Job drawing, mm, ordinate dimensions from the low corner. One solid piece. Give positions to 0.01 mm unless a question says otherwise; leave off trailing zeros. Write each loop counter-clockwise with the first axis right and the second up, starting at its lowest first coordinate (ties: lowest second). Pieces come first, ordered by that corner, then holes. Notation, with made-up numbers: (-18.75, 16) -> (1.25, 16) arc R22 cw to (1.25, 35) -> close; hole circle Ø2 at (-27.5, 83.25). An arc over 180 degrees is marked (long way). One line per question, with ' | ' between items. Start each with the question number.
(1) Band-saw the part on A-A, the plane z = 8. Give the cut face in (x, y).
(2) Band-saw the part on D-D, the plane x = 7. Give the cut face in (y, z), and give its area (3 significant figures).
(3) Pin check, flat tips, straight feed: P1, Ø2, axis at x = 4.5, y = 3.5, coming from the -Z side; P2, Ø2, axis at x = 32, y = 3.5, coming from the +Z side; P3, Ø4, axis at x = 11, z = 48, coming from the +Y side. Stop position of each tip, or through.
(4) Band-saw the part on C-C, the plane x = 11. Give the cut face in (y, z).
(5) Band-saw the part on B-B, the plane y = 1. Give the cut face in (x, z), and give its area (3 significant figures).
(6) Drill centre lines: probe 1 along Z at (x, y) = (27, 1.4); probe 2 along X at (y, z) = (0.45, 8); probe 3 along X at (y, z) = (3.75, 32). Where is each one in solid material? Low to high. Write a range as from..to.
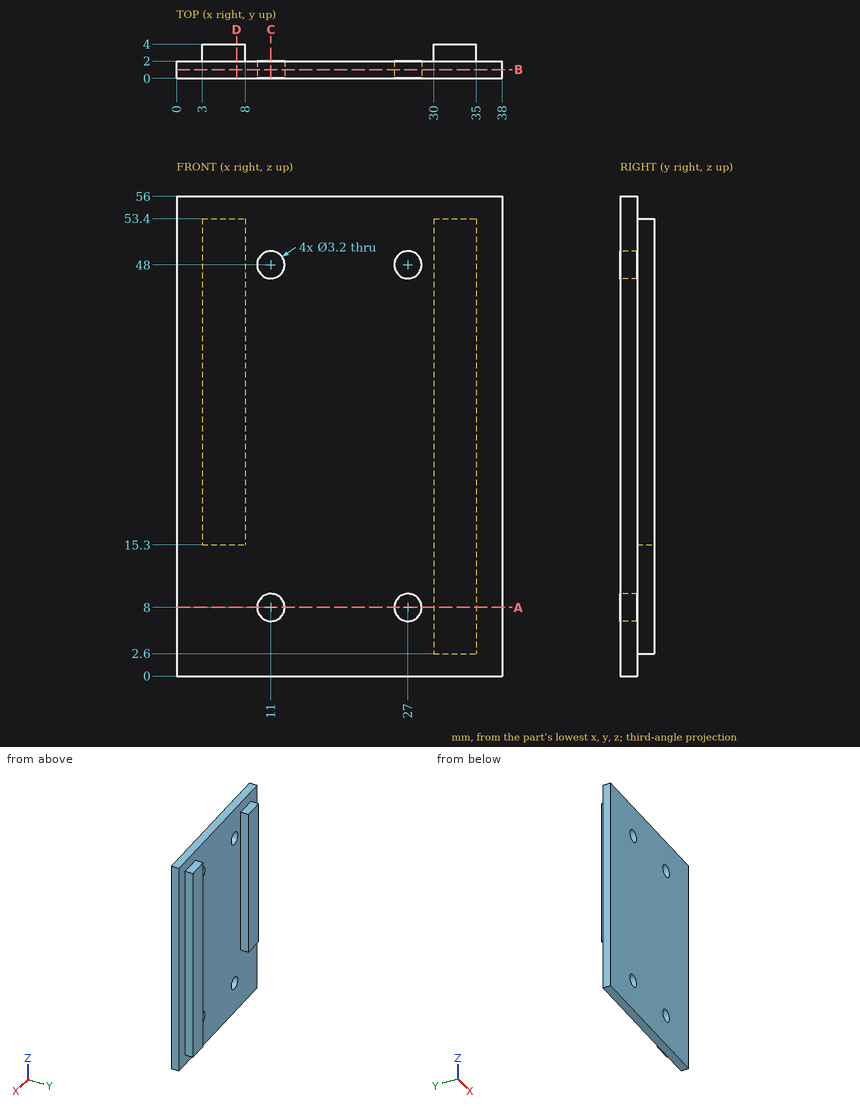
Results:
1) outline: (0, 0) -> (9.4, 0) -> (9.4, 2) -> (0, 2) -> close; (12.6, 0) -> (25.4, 0) -> (25.4, 2) -> (12.6, 2) -> close; (28.6, 0) -> (38, 0) -> (38, 2) -> (35, 2) -> (35, 4) -> (30, 4) -> (30, 2) -> (28.6, 2) -> close
2) outline: (0, 0) -> (2, 0) -> (2, 15.3) -> (4, 15.3) -> (4, 53.4) -> (2, 53.4) -> (2, 56) -> (0, 56) -> close | area: 188 mm²
3) P1: stops at z = 15.3 | P2: stops at z = 53.4 | P3: stops at y = 2
4) outline: (0, 0) -> (2, 0) -> (2, 6.4) -> (0, 6.4) -> close; (0, 9.6) -> (2, 9.6) -> (2, 46.4) -> (0, 46.4) -> close; (0, 49.6) -> (2, 49.6) -> (2, 56) -> (0, 56) -> close
5) outline: (0, 0) -> (38, 0) -> (38, 56) -> (0, 56) -> close; hole circle Ø3.2 at (11, 8); hole circle Ø3.2 at (11, 48); hole circle Ø3.2 at (27, 8); hole circle Ø3.2 at (27, 48) | area: 2,100 mm²
6) probe 1: z = 0..6.4, 9.6..46.4, 49.6..56 | probe 2: x = 0..9.4, 12.6..25.4, 28.6..38 | probe 3: x = 3..8, 30..35
